Geometry check sheet. Reference: the model listing, model coordinates, mm. A direction names the side the tool comes from. Round coordinates to 2 decimals unless told otherwise and drop trailing zeros. Order: outer loops, then holes, each group sorted by start corner. A loop starts at its lowest first (then second) coordinate and runs counter-clockwise, first axis right, second up. Notation, with made-up numbers: (38, 63) -> (43, 63) arc R20 ccw to (43, 80) -> close; hole circle Ø3 at (59, 89.25). An arc over 180 degrees is marked (long way). Answer as a JSON object with one key per item and string values. Group by question number.
from build123d import *

# Parameters (mm, degrees)
F0_W     = 6.35
F0_H     = 6.35
F0_W_2   = 12.7
F1_DEPTH = 6.35


# Not quite as in the source:
# - a feature names something its author has since deleted; it is built from what else it names


with BuildPart() as f1:
    # F0 (on Front) → F1 (new body)
    with BuildSketch(Plane.XZ):
        Polygon((38.1, 3.175), (38.1, 9.525), (-38.1, 9.525), (-38.1, 3.175), (-38.1, -3.175), (-34.925, -3.175), (-34.925, 3.175), (-15.875, 3.175), (-15.875, -3.175), (-12.7, -3.175), (0, -3.175), (12.7, -3.175), (15.875, -3.175), (15.875, 3.175), (34.925, 3.175), (34.925, -3.175), (38.1, -3.175), align=None)
        Polygon((-44.45, 3.175), (-44.45, 9.525), (-57.15, 9.525), (-57.15, 3.175), (-57.15, -3.175), (-44.45, -3.175), align=None)
        with Locations((-60.325, 0)):
            Rectangle(F0_W, F0_H)
        with Locations((-41.275, 0)):
            Rectangle(F0_W, F0_H)
        with Locations((41.275, 0)):
            Rectangle(F0_W, F0_H)
        with Locations((60.325, 0)):
            Rectangle(F0_W, F0_H)
        Polygon((57.15, 3.175), (57.15, 9.525), (44.45, 9.525), (44.45, 3.175), (44.45, -3.175), (57.15, -3.175), align=None)
        Polygon((-34.925, -3.175), (-38.1, -3.175), (-38.1, -9.525), (-25.4, -9.525), (-25.4, -3.175), align=None)
        with Locations((-6.35, -6.35)):
            Rectangle(F0_W_2, F0_H)
        Polygon((12.7, -9.525), (25.4, -9.525), (25.4, -3.175), (19.05, -3.175), (15.875, -3.175), (12.7, -3.175), align=None)
    extrude(amount=F1_DEPTH)


solid = f1.part
Item 1: Mould release check, pull along X, two halves, no side actions. Record for faces 6 (the flat face through (63.5, -3, 0)), 7 (the flat face through (-44.45, -3, 6)), 8 (the flat face through (-60, -3, 3.175)), 9 (the flat face through (-26, -3, 3.175)): pulls with the +X half, pulls with the -X half, needs draft (parallel to the pull), parting line crosses it, or undercut.
Item 2: Sectioned sample at A-A, the plane z = -6.25. Enter the section's corners in (x, y), then the cut area to 3 significant figures.
Item 3: Depth check by flat-ended pin: pin 1 Ø4 at (x, z) = (-18, -4.5) entering from +Y; pin 2 Ø1.9 at (y, z) = (-4, 5.5) entering from -X; pin 3 Ø3 at (y, z) = (-2, -5) entering from +X; pin 4 Ø2 at (y, z) = (-2, 5) entering from +X. Enter the tip coordinate at first touch or a pass-through.
Item 4: Sectioned sample at B-B, the plane x = 20.5. Enter the section's corners in (y, z) (3 decimals).
Item 5: Sectioned sample at D-D, the plane x = -18.5. Enter the section's corners in (y, z) (3 decimals), then the cut area to 3 significant figures.
Item 6: Thickness scan on L1, parallel to X at y = -5.5, z = -7; L2, parallel to X at y = -6, z = 7; L3, parallel to Z at x = 21.5, y = -5.25 (3 decimals). Record the ranges inside material, lowest first.
Item 7: Set-up check for faces 1 (the flat face through (-12.7, -3, -6)), 2 (the flat face through (60, -3, 3.175)), 3 (the flat face through (25, -3, 3.175)), 4 (the flat face through (38.1, -3, 6)), 5 (the flat face through (-51, -3, -3.175)): record each of +Z, -Z, +X, -X, +Y, -Y from which the full face is reachable in a straight line by a thin tool's end or side.
Item 8: Sectioned sample at C-C, the plane z = -1. Enter the section's corners in (x, y) (3 decimals).
Result:
{
 "1": {"face 6": "pulls with the +X half", "face 7": "undercut", "face 8": "needs draft", "face 9": "undercut"},
 "2": {"outline": "(-38.1, -6.35) -> (-25.4, -6.35) -> (-25.4, 0) -> (-38.1, 0) -> close; (-12.7, -6.35) -> (0, -6.35) -> (0, 0) -> (-12.7, 0) -> close; (12.7, -6.35) -> (25.4, -6.35) -> (25.4, 0) -> (12.7, 0) -> close", "area": "242 mm2"},
 "3": {"pin 1": "passes through", "pin 2": "stops at x = -57.15", "pin 3": "stops at x = 25.4", "pin 4": "stops at x = 57.15"},
 "4": {"outline": "(-6.35, -9.525) -> (0, -9.525) -> (0, -3.175) -> (-6.35, -3.175) -> close; (-6.35, 3.175) -> (0, 3.175) -> (0, 9.525) -> (-6.35, 9.525) -> close"},
 "5": {"outline": "(-6.35, 3.175) -> (0, 3.175) -> (0, 9.525) -> (-6.35, 9.525) -> close", "area": "40.3 mm2"},
 "6": {"L1": "x = -38.1 to -25.4, -12.7 to 0, 12.7 to 25.4", "L2": "x = -57.15 to -44.45, -38.1 to 38.1, 44.45 to 57.15", "L3": "z = -9.525 to -3.175, 3.175 to 9.525"},
 "7": {"face 1": "-Z, +Y, -Y", "face 2": "+Z, +X, +Y, -Y", "face 3": "+Y, -Y", "face 4": "+Z, +Y, -Y", "face 5": "-Z, -X, +Y, -Y"},
 "8": {"outline": "(-63.5, -6.35) -> (-34.925, -6.35) -> (-34.925, 0) -> (-63.5, 0) -> close; (-15.875, -6.35) -> (15.875, -6.35) -> (15.875, 0) -> (-15.875, 0) -> close; (34.925, -6.35) -> (63.5, -6.35) -> (63.5, 0) -> (34.925, 0) -> close"}
}
